```python
from build123d import *

# Parameters (mm, degrees)
SKETCH1_W               = 180
SKETCH1_H               = 350
BOSS_EXTRUDE1_DEPTH     = 100
SKETCH2_R               = 75
BOSS_EXTRUDE2_DEPTH     = 450
SKETCH3_W               = 45.419423784
SKETCH3_H               = 142.958301414
BOSS_EXTRUDE3_DEPTH     = 200
FILLET1_R               = 80
CUT_EXTRUDE1_DEPTH      = 778.911353606
CUT_EXTRUDE1_DEPTH_BACK = 778.911353606
SKETCH4_R               = 19.812422485


with BuildPart() as part:
    # Sketch1 → Boss-Extrude1 (new body)
    with BuildSketch(Plane(origin=(0, 0, 0), x_dir=(1, 0, 0), z_dir=(0, 1, 0))):
        Rectangle(SKETCH1_W, SKETCH1_H)
    extrude(amount=BOSS_EXTRUDE1_DEPTH)

    # Sketch2 → Boss-Extrude2 (add)
    with BuildSketch(Plane(origin=(0, 100, 0), x_dir=(1, 0, 0), z_dir=(0, 1, 0))):
        with Locations(Location((0, 100, 0), (0, 0, 90))):
            Circle(SKETCH2_R)
    extrude(amount=BOSS_EXTRUDE2_DEPTH)

    # Sketch3 → Boss-Extrude3 (add)
    with BuildSketch(Plane(origin=(0, 550, 0), x_dir=(1, 0, 0), z_dir=(0, 1, 0))):
        with Locations((0, 100)):
            Rectangle(SKETCH3_W, SKETCH3_H)
    extrude(amount=BOSS_EXTRUDE3_DEPTH)

    # Fillet1
    # the kernel refuses this fillet: 80 mm, written as the material it takes off along each edge
    with BuildSketch(Plane(origin=(222.709711892, 750, -171.479150707), x_dir=(0, -1, 0), z_dir=(-1, 0, 0)), Plane(origin=(-222.709711892, 750, -28.520849293), x_dir=(0, -1, 0), z_dir=(1, 0, 0))) as fillet1_piece_1:
        with BuildLine():
            CenterArc((FILLET1_R, FILLET1_R), FILLET1_R, 180, 90)
            Line((0, FILLET1_R), (0, 0))
            Line((0, 0), (FILLET1_R, 0))
        make_face()
    extrude(amount=445.419423783, mode=Mode.SUBTRACT)

    # Sketch4 → Cut-Extrude1 (cut, two sides: drawn at the far end of the back side and taken through both)
    with BuildSketch(Plane(origin=(-22.709711892, 0, 0), x_dir=(0, 0, -1), z_dir=(1, 0, 0)).offset(-CUT_EXTRUDE1_DEPTH_BACK)):
        with Locations((100, 649.772462607)):
            Circle(SKETCH4_R)
    extrude(amount=CUT_EXTRUDE1_DEPTH + CUT_EXTRUDE1_DEPTH_BACK, mode=Mode.SUBTRACT)


solid = part.part
```
Here's how the part is built. I have some questions about the finished solid (model axes, mm). A direction names the side the tool comes from. Give positions to 0.01 mm unless a question says otherwise; leave off trailing zeros. Order: outer loops, then holes, each group sorted by start corner. A loop starts at its lowest first (then second) coordinate and runs counter-clockwise, first axis right, second up. Notation, with made-up numbers: (87, 17) - (111, 17) arc R21 cw to (111, 45) - close; hole circle Ø11 at (31, 89). An arc over 180 degrees is marked (long way). Answer as a JSON object with one key per item and string values. Group by question number.
Item 1: Which directions (+Z, -Z, +X, -X, +Y, -Y) give clear straight access to the entire face, cutting with the end or side of a thin tool? Please do faces 4 (the cylindrical face through (-22.528, 321.85, -171.537)), 5 (the flat face through (0, 609, -28.521)), 6 (the flat face through (-22.71, 626, -99)).
Item 2: If we section it at D-D on x = -65: Please give me the cut outline in (y, z).
Item 3: For P1, Ø12, axis at x = -13, y = 222.5, coming from the +Z side; P2, Ø10, axis at x = -5.5, y = 505.5, coming from the -Z side; P3, Ø3, axis at y = 636.5, z = -40, coming from the -X side, each with a flat end and sliding along its axis, tell me the tip position at first contact or that it passes through.
Item 4: If we section it at B-B on x = 39.5: Please give me the cut outline in (y, z), and give its area (3 significant figures).
Item 5: Please list where these lines run through material, in increasing order: probe 1 along Z at (x, y) = (-4.5, 556); probe 2 along Z at (x, y) = (2, 453); probe 3 along Y at (x, z) = (-19, -5).
Item 6: If we mould it in two halves opening along Y, with no side actions, what happens to faces 1 (the cylindrical face through (-0.318, 632.195, -109.142)), 2 (the flat face through (22.71, 626, -99)), 3 (the flat face through (-1, 100, 36))? For each: pulls with the +Y half, pulls with the -Y half, needs draft (parallel to the pull), parting line crosses it, or undercut.
Item 7: If we section it at C-C on y = 367: Please give me the cut outline in (x, z), and give its area (3 significant figures).
Item 8: If we section it at A-A on z = -111.5: Please give me the cut outline in (x, y).
Result set:
{
 "1": {"face 4": "+Y", "face 5": "+Z, +X, -X, +Y", "face 6": "+Z, -Z, -X, +Y"},
 "2": {"outline": "(0, -175) - (100, -175) - (100, -137.42) - (550, -137.42) - (550, -62.58) - (100, -62.58) - (100, 175) - (0, 175) - close"},
 "3": {"P1": "z = -25.33", "P2": "z = -175", "P3": "x = -22.71"},
 "4": {"outline": "(0, -175) - (100, -175) - (100, -163.76) - (550, -163.76) - (550, -36.24) - (100, -36.24) - (100, 175) - (0, 175) - close", "area": "92,400 mm²"},
 "5": {"probe 1": "-171.48 to -28.52", "probe 2": "-174.97 to -25.03", "probe 3": "0 to 100"},
 "6": {"face 1": "undercut", "face 2": "needs draft", "face 3": "pulls with the +Y half"},
 "7": {"outline": "circle Ø150 at (0, -100)", "area": "17,700 mm²"},
 "8": {"outline": "(-90, 0) - (90, 0) - (90, 100) - (74.11, 100) - (74.11, 550) - (22.71, 550) - (22.71, 633.64) - (-22.71, 633.64) - (-22.71, 550) - (-74.11, 550) - (-74.11, 100) - (-90, 100) - close; (-22.71, 665.91) - (22.71, 665.91) - (22.71, 747.45) - (-22.71, 747.45) - close"}
}
